Design review of the part built by this model. Coordinates are the model's own, in mm. A direction names the side the tool comes from. Round coordinates to 2 decimals unless told otherwise and drop trailing zeros. Loops run counter-clockwise (first coordinate to the right, second up) from the corner with the lowest first, then second, coordinate; pieces in that order, holes last. Notation, with made-up numbers: M 33.5,84.5 L 52.5,84.5 A29 ccw 52.5,104.5 Z; hole C 48,86.25 d9. An arc over 180 degrees is marked long. Use a Markdown table: item, result.
from build123d import *

# Parameters (mm, degrees)
SKETCH1_R           = 52
SKETCH1_R_2         = 33
BOSS_EXTRUDE1_DEPTH = 3.3
SKETCH2_R           = 35
SKETCH2_R_2         = 33
BOSS_EXTRUDE2_DEPTH = 27
SKETCH3_R           = 2.25
CUT_EXTRUDE1_DEPTH  = 4.3
CIRPATTERN1_COUNT   = 12


with BuildPart() as part:
    # Sketch1 → Boss-Extrude1 (new body)
    with BuildSketch(Plane(origin=(0, 0, 0), x_dir=(1, 0, 0), z_dir=(0, 1, 0))):
        Circle(SKETCH1_R)
        Circle(SKETCH1_R_2, mode=Mode.SUBTRACT)
    extrude(amount=BOSS_EXTRUDE1_DEPTH)

    # Sketch2 → Boss-Extrude2 (add)
    with BuildSketch(Plane(origin=(0, 3.3, 0), x_dir=(1, 0, 0), z_dir=(0, 1, 0))):
        Circle(SKETCH2_R)
        Circle(SKETCH2_R_2, mode=Mode.SUBTRACT)
    extrude(amount=BOSS_EXTRUDE2_DEPTH)

    # Sketch3 → Cut-Extrude1 (cut, through all)
    with BuildSketch(Plane(origin=(0, 3.3, 0), x_dir=(1, 0, 0), z_dir=(0, 1, 0))):
        with Locations((0, 48)):
            Circle(SKETCH3_R)
    cut_extrude1 = extrude(amount=-CUT_EXTRUDE1_DEPTH, mode=Mode.SUBTRACT)

    # CirPattern1: Cut-Extrude1 ×12 about axis
    cirpattern1_axis = Axis((0, 0, 0), (0, 1, 0))
    for i in range(1, CIRPATTERN1_COUNT):
        add(cut_extrude1.rotate(cirpattern1_axis, i * 360 / CIRPATTERN1_COUNT), mode=Mode.SUBTRACT)


solid = part.part
1. Take a section at D-D on z = 24. Give the boundary of the cut face in (x, y).
Check values:
| item | result |
|---|---|
| outline | M -46.13,0 L -43.82,0 L -43.82,3.3 L -46.13,3.3 Z; M -39.32,0 L -22.65,0 L -22.65,30.3 L -25.48,30.3 L -25.48,3.3 L -39.32,3.3 Z; M 22.65,0 L 39.32,0 L 39.32,3.3 L 25.48,3.3 L 25.48,30.3 L 22.65,30.3 Z; M 43.82,0 L 46.13,0 L 46.13,3.3 L 43.82,3.3 Z |
2. Take a section at C-C on x = -48. Give the boundary of the cut face in (y, z), and give its area (3 significant figures).
Check values:
| item | result |
|---|---|
| outline | M 0,-20 L 3.3,-20 L 3.3,-2.25 L 0,-2.25 Z; M 0,2.25 L 3.3,2.25 L 3.3,20 L 0,20 Z |
| area | 117 mm² |
3. Insertion check: pin 1 (4 mm diameter, centred on x = 38, z = -33.5, fed in from +Y); pin 2 (3 mm diameter, centred on x = -21, y = 22, fed in from +Z); pin 3 (2 mm diameter, centred on y = 14, z = -17.5, fed in from -X). Each pin has a flat end and moves straight along its axis. Give the tip position at first contact, or say it passes through.
Check values:
| item | result |
|---|---|
| pin 1 | stops at y = 3.3 |
| pin 2 | stops at z = 29.06 |
| pin 3 | stops at x = -30.87 |
4. Take a section at B-B on x = 0. Give the boundary of the cut face in (y, z).
Check values:
| item | result |
|---|---|
| outline | M 0,-52 L 3.3,-52 L 3.3,-50.25 L 0,-50.25 Z; M 0,-45.75 L 3.3,-45.75 L 3.3,-35 L 30.3,-35 L 30.3,-33 L 0,-33 Z; M 0,33 L 30.3,33 L 30.3,35 L 3.3,35 L 3.3,45.75 L 0,45.75 Z; M 0,50.25 L 3.3,50.25 L 3.3,52 L 0,52 Z |
5. Machinability: for faces 1 (the face through (-41.265, 1.627, 31.641)), 2 (the face through (11, 3.3, 34)), which of the approach directions +Z, -Z, +X, -X, +Y, -Y give a long, thin tool a straight path to every point of the face, cutting with its end or side? Answer none if there is none.
Check values:
| item | result |
|---|---|
| face 1 | +Y, -Y |
| face 2 | +Y |
6. Take a section at A-A on z = -48. Give the boundary of the cut face in (x, y).
Check values:
| item | result |
|---|---|
| outline | M -20,0 L -2.25,0 L -2.25,3.3 L -20,3.3 Z; M 2.25,0 L 20,0 L 20,3.3 L 2.25,3.3 Z |
7. Wall thickness on line 1 along Z through (x, y) = (0, 1.5); line 2 along X through (y, z) = (20, -20.5): over which ranges is each line inside the solid? List them lowest first. Write a range as from..to.
Check values:
| item | result |
|---|---|
| line 1 | z = -52..-50.25, -45.75..-33, 33..45.75, 50.25..52 |
| line 2 | x = -28.37..-25.86, 25.86..28.37 |
8. The part is to be moulded in two halves that separate along Z. For faces 3 (the face through (30.5, 14.9, 12.6)), 4 (the face through (-23.5, 30.3, -23.5)), 5 (the face through (-28, 17, 21)), say which applies: pulls with the +Z half, pulls with the -Z half, needs draft (parallel to the pull), parting line crosses it, or undercut.
Check values:
| item | result |
|---|---|
| face 3 | undercut |
| face 4 | needs draft |
| face 5 | parting line crosses it |
